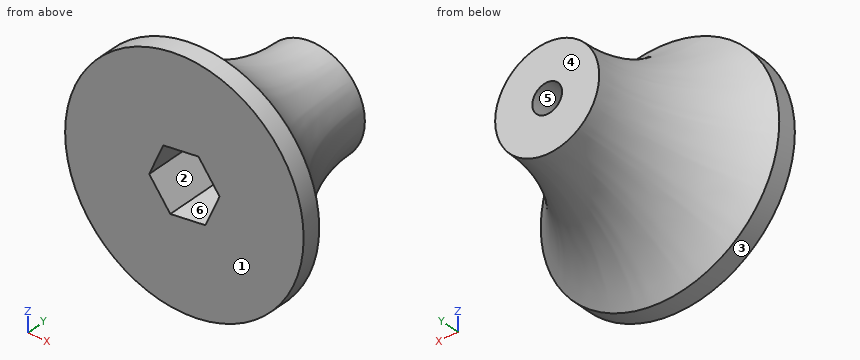
from build123d import *

# Parameters (mm, degrees)
CUT_EXTRUDE1_DEPTH = 16.096219


with BuildPart() as part:
    # Sketch2 → Revolve1 (revolve)
    with BuildSketch(Plane.XY):
        with BuildLine():
            Line((2.032, -2.634219297), (2.032, 19.05))
            Line((2.032, 19.05), (7.112, 19.05))
            ThreePointArc((7.112, 19.05), (9.527739154, 8.475956955), (16.295629201, 0))
            Line((16.295629201, 0), (16.295629201, -2.634219297))
            Line((16.295629201, -2.634219297), (2.032, -2.634219297))
        make_face()
    revolve(axis=Axis((0, 0, 0), (0, 1, 0)))

    # Sketch3 → Cut-Extrude1 (cut)
    with BuildSketch(Plane.XZ.offset(2.634219297)):
        Polygon((4.80775348, 0.552100056), (1.925744066, 4.439686677), (-2.882009414, 3.887586621), (-4.80775348, -0.552100056), (-1.925744066, -4.439686677), (2.882009414, -3.887586621), align=None)
    extrude(amount=-CUT_EXTRUDE1_DEPTH, mode=Mode.SUBTRACT)


solid = part.part
CAD build for the part. Positions are in the model's coordinates, mm. Face numbers are marked on the shaded views. A direction names the side the tool comes from. Coordinates: 2 decimals unless noted, no trailing zeros. Order: outer loops, then holes, each group sorted by start corner. A loop starts at its lowest first (then second) coordinate and runs counter-clockwise, first axis right, second up. Notation, with made-up numbers: (59.5, 44.5) -> (117.5, 44.5) arc R11 cw to (117.5, 59.5) -> close; hole circle Ø6 at (15.25, -1.5). An arc over 180 degrees is marked (long way). Answer in a Markdown table with one row per item.
1) Band-saw the part on A-A (x = 0). List the corners of the cut face in (y, z).
Check values:
| item | result |
|---|---|
| outline | (-2.63, -16.3) -> (0, -16.3) arc R24.35 cw to (19.05, -7.11) -> (19.05, -2.03) -> (13.46, -2.03) -> (13.46, -4.22) -> (-2.63, -4.22) -> close; (-2.63, 4.22) -> (13.46, 4.22) -> (13.46, 2.03) -> (19.05, 2.03) -> (19.05, 7.11) arc R24.35 cw to (0, 16.3) -> (-2.63, 16.3) -> close |
2) Band-saw the part on B-B (y = 1). List the corners of the cut face in (x, z).
Check values:
| item | result |
|---|---|
| outline | circle Ø30.24 at (0, 0); hole (-4.81, -0.55) -> (-1.93, -4.44) -> (2.88, -3.89) -> (4.81, 0.55) -> (1.93, 4.44) -> (-2.88, 3.89) -> close |
3) Band-saw the part on C-C (z = 0). List the corners of the cut face in (x, y).
Check values:
| item | result |
|---|---|
| outline | (-16.3, -2.63) -> (-4.57, -2.63) -> (-4.57, 13.46) -> (-2.03, 13.46) -> (-2.03, 19.05) -> (-7.11, 19.05) arc R24.35 cw to (-16.3, 0) -> close; (2.03, 13.46) -> (4.57, 13.46) -> (4.57, -2.63) -> (16.3, -2.63) -> (16.3, 0) arc R24.35 cw to (7.11, 19.05) -> (2.03, 19.05) -> close |
4) Which spindle directions (+Z, -Z, +X, -X, +Y, -Y) get a long thin tool onto all of the face, cutting with end or side? Do the marked faces 1 and 2. Say none if no direction does.
Check values:
| item | result |
|---|---|
| face 1 | +Z, -Z, +X, -X, -Y |
| face 2 | -Y |
5) Drill centre lines: line 1 (X direction, y = 17.45, z = 0); line 2 (Z direction, x = 0, y = 15.85); line 3 (Z direction, x = 4, y = 4.25). Where is each one in solid material? Low to high.
Check values:
| item | result |
|---|---|
| line 1 | -7.16 to -2.03, 2.03 to 7.16 |
| line 2 | -7.32 to -2.03, 2.03 to 7.32 |
| line 3 | -11.45 to -1.31, 1.64 to 11.45 |
6) Mould opens along X. For the marked faces 3, 4, 5 and 6 say: pulls with the +X half, pulls with the -X half, needs draft (parallel to the pull), parting line crosses it, or undercut.
Check values:
| item | result |
|---|---|
| face 3 | parting line crosses it |
| face 4 | needs draft |
| face 5 | undercut |
| face 6 | undercut |
7) Band-saw the part on D-D (y = 15). List the corners of the cut face in (x, z), and give its area (3 significant figures).
Check values:
| item | result |
|---|---|
| outline | circle Ø14.9 at (0, 0); hole circle Ø4.06 at (0, 0) |
| area | 161 mm2 |
8) Flat gauge pins, fed straight in: P1, Ø10, axis at x = 0, z = 0, coming from the -Y side; P2, Ø6, axis at y = 5.5, z = 4, coming from the -X side; P3, Ø10, axis at x = -10.5, y = 7, coming from the +Z side; P4, Ø1.5, axis at x = -4.5, z = 10.5, coming from the +Y side. Where does each tip first touch, or does it go through?
Check values:
| item | result |
|---|---|
| P1 | y = -2.63 |
| P2 | x = -13.12 |
| P3 | z = 10.82 |
| P4 | y = 6.37 |
